Geometry: final body of the model. Coordinates: model frame, mm. A direction names the side the tool comes from. Give positions to 0.01 mm unless a question says otherwise; leave off trailing zeros. Write each loop counter-clockwise with the first axis right and the second up, starting at its lowest first coordinate (ties: lowest second). Pieces come first, ordered by that corner, then holes. Notation, with made-up numbers: M -40,37.5 L 7,37.5 A28 cw 7,68.5 Z; hole C 20.25,82.5 d1. An arc over 180 degrees is marked long. Use a Markdown table: item, result. Add a question column.
(1) Cut plane A-A (z = 4.35). Output: boundary loops of the cut face in (x, y), plus the area to 3 significant figures.
(2) Cut plane B-B (y = -9). Output: boundary loops of the cut face in (x, z).
(3) Pin query (flat end, axial travel): pin 1 Ø1.5 at (y, z) = (-14.5, 1.5) entering from +X; pin 2 Ø1.8 at (x, z) = (-26.5, 3) entering from +Y; pin 3 Ø3 at (x, z) = (-16.5, 2.5) entering from +Y. Return the tip coordinate at first contact, or that it passes through.
(4) Cut plane C-C (y = 20.5). Output: boundary loops of the cut face in (x, z), plus the area to 3 significant figures.
(5) Reachability of faces 1 (the flat face through (-22.267, -7, 3)), 2 (the flat face through (31, -0.933, 3)), 3 (the flat face through (31, 7.067, 3)), 4 (the flat face through (-25, 8.067, 3)) from +Z, -Z, +X, -X, +Y, -Y: full face, straight path, thin tool, end or side. Return the list, or none.
(6) Material intervals for L1, parallel to X at y = -10, z = 0.45; L2, parallel to Y at x = -9, z = 3.4; L3, parallel to X at y = 22, z = 2.3, sorted ascending.
```python
from build123d import *

# Parameters (mm, degrees)
ESQUISSE1_W        = 50
ESQUISSE1_H        = 30
BOSS_EXTRU_1_DEPTH = 6
ESQUISSE3_W        = 30
ESQUISSE3_H        = 8
BOSS_EXTRU_2_DEPTH = 6
CONG_1_R           = 10
CONG_2_R           = 10
CONG_3_R           = 10
CONG_4_R           = 10
ESQUISSE7_W        = 6
ESQUISSE7_H        = 10
ESQUISSE7_H_2      = 8
BOSS_EXTRU_3_DEPTH = 6


with BuildPart() as part:
    # Esquisse1 → Boss.-Extru.1 (new body)
    with BuildSketch(Plane.XY):
        with Locations((2.73294214, 3.066688104)):
            Rectangle(ESQUISSE1_W, ESQUISSE1_H)
    extrude(amount=BOSS_EXTRU_1_DEPTH)

    # Esquisse3 → Boss.-Extru.2 (add)
    with BuildSketch(Plane.XY.offset(6)):
        with Locations((12.73294214, 22.066688104)):
            Rectangle(ESQUISSE3_W, ESQUISSE3_H)
        with Locations((12.73294214, -15.933311896)):
            Rectangle(ESQUISSE3_W, ESQUISSE3_H)
    extrude(amount=-BOSS_EXTRU_2_DEPTH)

    # Congé1
    # the kernel refuses this fillet: 10 mm, written as the material it takes off along each edge
    with BuildSketch(Plane(origin=(-2.26705786, 26.066688104, 30.494897428), x_dir=(1, 0, 0), z_dir=(0, 0, -1))) as cong_1_piece_1:
        with BuildLine():
            CenterArc((9.797958971, 10), CONG_1_R, 191.536959033, 78.463040967)
            Line((0, 8), (-0.195959179, 7.96))
            ThreePointArc((-0.195959179, 7.96), (-0.2, 4), (-0.2, 0))
            Line((-0.2, 0), (0, -0.2))
            Line((0, -0.2), (9.797958971, -0.2))
            Line((9.797958971, -0.2), (9.797958971, 0))
        make_face()
    extrude(amount=54.989794856, mode=Mode.SUBTRACT)

    # Congé2
    # the kernel refuses this fillet: 10 mm, written as the material it takes off along each edge
    with BuildSketch(Plane(origin=(-2.26705786, -19.933311896, 30.494897428), x_dir=(0, 1, 0), z_dir=(0, 0, -1))) as cong_2_piece_1:
        with BuildLine():
            CenterArc((10, 9.797958971), CONG_2_R, 180, 78.463040967)
            Line((0, 9.797958971), (-0.2, 9.797958971))
            Line((-0.2, 9.797958971), (-0.2, 0))
            Line((-0.2, 0), (0, -0.2))
            ThreePointArc((0, -0.2), (4, -0.2), (7.96, -0.195959179))
            Line((7.96, -0.195959179), (8, 0))
        make_face()
    extrude(amount=54.989794856, mode=Mode.SUBTRACT)

    # Congé3
    cong_3_edges = [part.edges().sort_by_distance(p)[0] for p in [
        (-2.26705786, 18.066688104, 3),
    ]]
    fillet(cong_3_edges, radius=CONG_3_R)

    # Congé4
    cong_4_edges = [part.edges().sort_by_distance(p)[0] for p in [
        (-2.26705786, -11.933311896, 3),
    ]]
    fillet(cong_4_edges, radius=CONG_4_R)

    # Esquisse7 → Boss.-Extru.3 (add)
    with BuildSketch(Plane.XY.offset(6)):
        with Locations((-25.26705786, 3.066688104)):
            Rectangle(ESQUISSE7_W, ESQUISSE7_H)
        with Locations((30.73294214, 3.066688104)):
            Rectangle(ESQUISSE7_W, ESQUISSE7_H_2)
    extrude(amount=-BOSS_EXTRU_3_DEPTH)


solid = part.part
```
Answer list:
| question | item | result |
|---|---|---|
| 1 | outline | M -28.27,-1.93 L -22.27,-1.93 L -22.27,-11.93 L -8.47,-11.93 A10 cw -0.47,-15.93 A10 ccw 7.53,-19.93 L 27.73,-19.93 L 27.73,-0.93 L 33.73,-0.93 L 33.73,7.07 L 27.73,7.07 L 27.73,26.07 L 7.53,26.07 A10 ccw -0.47,22.07 A10 cw -8.47,18.07 L -22.27,18.07 L -22.27,8.07 L -28.27,8.07 Z |
| 1 | area | 2,060 mm² |
| 2 | outline | M -22.27,0 L 27.73,0 L 27.73,6 L -22.27,6 Z |
| 3 | pin 1 | x = 27.73 |
| 3 | pin 2 | y = 8.07 |
| 3 | pin 3 | y = 18.07 |
| 4 | outline | M -1.93,0 L 27.73,0 L 27.73,6 L -1.93,6 Z |
| 4 | area | 178 mm² |
| 5 | face 1 | +Z, -Z, -X, -Y |
| 5 | face 2 | +Z, -Z, +X, -Y |
| 5 | face 3 | +Z, -Z, +X, +Y |
| 5 | face 4 | +Z, -Z, -X, +Y |
| 6 | L1 | -22.27 to 27.73 |
| 6 | L2 | -11.93 to 18.07 |
| 6 | L3 | -0.52 to 27.73 |
